Build history of the part. All positions in model axes, mm. Face numbers are marked on the shaded views. A direction names the side the tool comes from. Round coordinates to 2 decimals unless told otherwise and drop trailing zeros. Write each loop counter-clockwise with the first axis right and the second up, starting at its lowest first coordinate (ties: lowest second). Pieces come first, ordered by that corner, then holes. Notation, with made-up numbers: M 56,81 L 108,81 A21 ccw 108,120 Z; hole C 11,49.5 d4. An arc over 180 degrees is marked long. One line per item, written item: value. Start each with the question number.
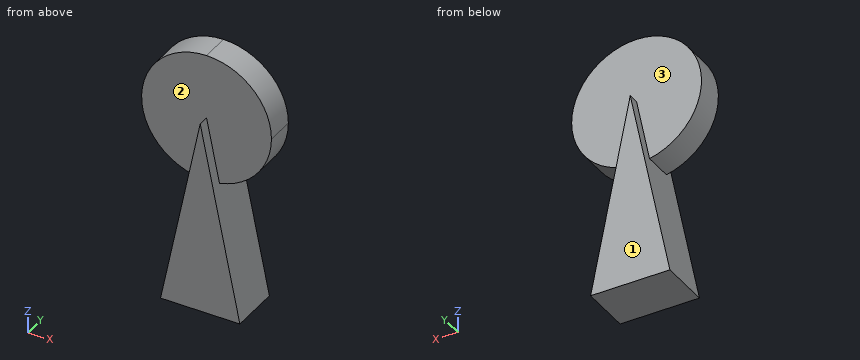
```python
from build123d import *

# Parameters (mm, degrees)
F1_DEPTH = 2
F3_DEPTH = 3.5


with BuildPart() as f1:
    # F0 (on Front) → F1 (new body, symmetric)
    with BuildSketch(Plane.XZ):
        with BuildLine():
            Line((0, 18), (0, 36))
            ThreePointArc((0, 36), (-9, 27), (0, 18))
        make_face()
        with BuildLine():
            ThreePointArc((0, 18), (6.363961, 20.636039), (9, 27))
            ThreePointArc((9, 27), (6.363961, 33.363961), (0, 36))
            Line((0, 36), (0, 18))
        make_face()
    extrude(amount=F1_DEPTH, both=True)

    # F2 (on Front) → F3 (join, symmetric)
    with BuildSketch(Plane.XZ):
        Polygon((5.5, 0), (0, 27), (-5.5, 0), align=None)
    extrude(amount=F3_DEPTH, both=True)

    # F4: F1 across plane


with BuildPart() as f1_1:
    add(f1.part)
    add(f1.part.mirror(Plane.XZ))


solid = f1_1.part
```
Item 1: Cut at B-B, the plane z = 19. Write the cut outline in (x, y), plus the area to 3 significant figures.
Item 2: Cut at C-C, the plane y = -1. Write the cut outline in (x, z).
Item 3: Which spindle directions (+Z, -Z, +X, -X, +Y, -Y) get a long thin tool onto all of the face, cutting with end or side? Do the marked faces 1, 2 and 3. Say none if no direction does.
Item 4: Drill centre lines: line 1 (Z direction, x = 0.25, y = -0.25); line 2 (Y direction, x = -1.75, z = 26); line 3 (Z direction, x = 6.5, y = 0). Where is each one in solid material? Low to high.
Item 5: Cut at D-D, the plane x = 1.25. Write the cut outline in (y, z), plus the area to 3 significant figures.
Item 6: Cut at A-A, the plane x = -3.25. Write the cut outline in (y, z).
Item 7: Drop a flat-ended pin along its axis: pin 1 (2 mm diameter, centred on y = 1, z = 20.5, fed in from +X). Give the stop position or say it passes through.
Computed values:
1. outline: M -4.12,-2 L -1.63,-2 L -1.63,-3.5 L 1.63,-3.5 L 1.63,-2 L 4.12,-2 L 4.12,2 L 1.63,2 L 1.63,3.5 L -1.63,3.5 L -1.63,2 L -4.12,2 Z
1. area: 42.8 mm2
2. outline: M -5.5,0 L 5.5,0 L 1.8,18.18 A9 ccw long -1.8,18.18 Z
3. face 1: +Z, -Z, +X, -X, +Y
3. face 2: +Z, -Y
3. face 3: +Z, +Y
4. line 1: z = 0 to 36
4. line 2: y = -2 to 2
4. line 3: z = 20.78 to 33.22
5. outline: M -3.5,0 L 3.5,0 L 3.5,20.86 L 2,20.86 L 2,35.91 L -2,35.91 L -2,20.86 L -3.5,20.86 Z
5. area: 206 mm2
6. outline: M -3.5,0 L 3.5,0 L 3.5,11.05 L -3.5,11.05 Z; M -2,18.61 L 2,18.61 L 2,35.39 L -2,35.39 Z
7. pin 1: stops at x = 7.12
